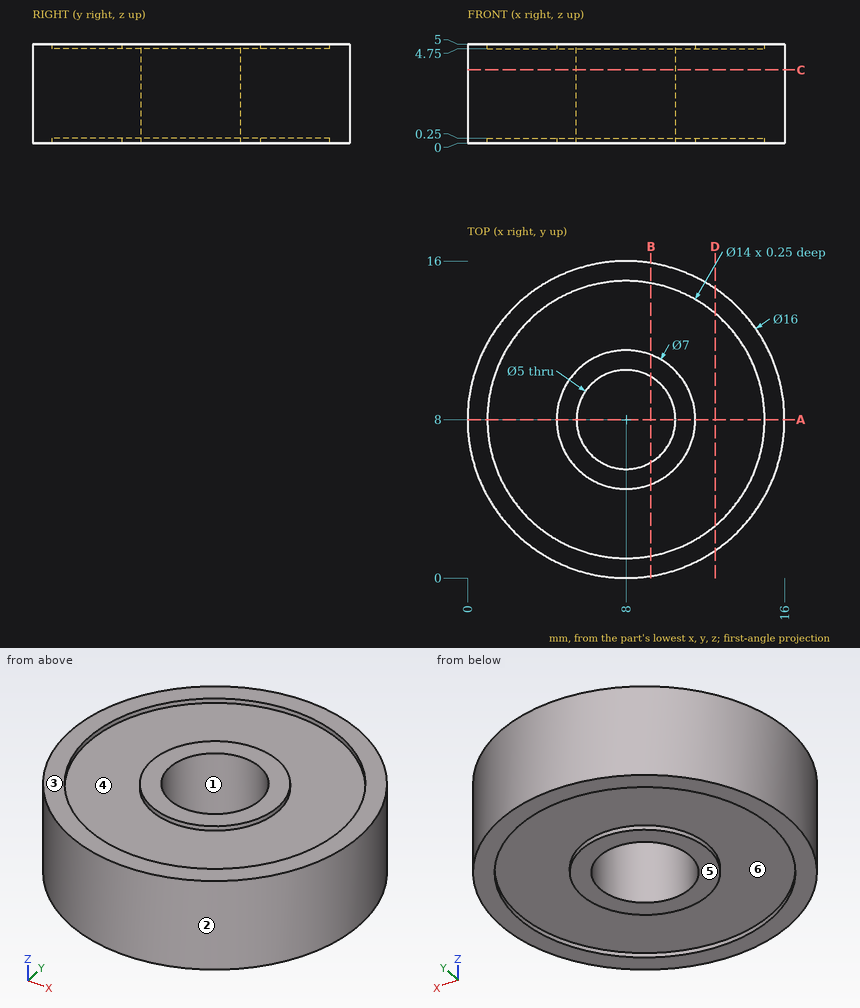
The figure shows three views and two pictorial views of one solid part (mm, origin at its lowest corner). Answer the questions. A direction names the side the tool comes from. Coordinates: 2 decimals unless noted, no trailing zeros. Order: outer loops, then holes, each group sorted by start corner. A loop starts at its lowest first (then second) coordinate and runs counter-clockwise, first axis right, second up. Notation, with made-up numbers: (-5.75, 16.5) - (20.25, 16.5) arc R16 ccw to (20.25, 20.5) - close; hole circle Ø8 at (-2.75, -23.75). An arc over 180 degrees is marked (long way). Answer as a JSON object with one key per item and string values.
1. Each of these flat-tipped pins is pushed along its axis until it touches: P1, Ø1.5, axis at x = 2.5, z = 0.5, coming from the +Y side; P2, Ø1, axis at x = 11.5, z = 0.5, coming from the -Y side. Where does it stop, or does it pass through?
Output values:
{"P1": "stops at y = 14.44", "P2": "stops at y = 0.58"}
2. Find section D-D on x = 12.5. Determine the outline of the cut face in (y, z), plus the area to 3 significant figures.
Output values:
{"outline": "(1.39, 0) - (2.64, 0) - (2.64, 0.25) - (13.36, 0.25) - (13.36, 0) - (14.61, 0) - (14.61, 5) - (13.36, 5) - (13.36, 4.75) - (2.64, 4.75) - (2.64, 5) - (1.39, 5) - close", "area": "60.8 mm²"}
3. Consider line 1 (X direction, y = 8, z = 0.1); line 2 (Y direction, x = 8, z = 2.9). Determine where each line is inside the solid, lowest interval first.
Output values:
{"line 1": "x = 0 to 1, 4.5 to 5.5, 10.5 to 11.5, 15 to 16", "line 2": "y = 0 to 5.5, 10.5 to 16"}
4. Find section A-A on y = 8. Determine the outline of the cut face in (x, z).
Output values:
{"outline": "(0, 0) - (1, 0) - (1, 0.25) - (4.5, 0.25) - (4.5, 0) - (5.5, 0) - (5.5, 5) - (4.5, 5) - (4.5, 4.75) - (1, 4.75) - (1, 5) - (0, 5) - close; (10.5, 0) - (11.5, 0) - (11.5, 0.25) - (15, 0.25) - (15, 0) - (16, 0) - (16, 5) - (15, 5) - (15, 4.75) - (11.5, 4.75) - (11.5, 5) - (10.5, 5) - close"}
5. The mould has two halves that part along X. Classify the marked faces 1, 2, 3 and 4: +X half, -X half, draft (parallel to the pull), parting line (faces both ways), or undercut.
Output values:
{"face 1": "undercut", "face 2": "parting line", "face 3": "draft", "face 4": "undercut"}
6. Find section B-B on x = 9.25. Determine the outline of the cut face in (y, z).
Output values:
{"outline": "(0.1, 0) - (1.11, 0) - (1.11, 0.25) - (4.73, 0.25) - (4.73, 0) - (5.83, 0) - (5.83, 5) - (4.73, 5) - (4.73, 4.75) - (1.11, 4.75) - (1.11, 5) - (0.1, 5) - close; (10.17, 0) - (11.27, 0) - (11.27, 0.25) - (14.89, 0.25) - (14.89, 0) - (15.9, 0) - (15.9, 5) - (14.89, 5) - (14.89, 4.75) - (11.27, 4.75) - (11.27, 5) - (10.17, 5) - close"}
7. Find section C-C on z = 3.7. Determine the outline of the cut face in (x, y).
Output values:
{"outline": "circle Ø16 at (8, 8); hole circle Ø5 at (8, 8)"}
8. A tool of negligible diameter and unlimited length cuts with its end or side. For the marked faces 5 and 6, from which of +Z, -Z, +X, -X, +Y, -Y can it reach the whole face along a straight path? Write none if from no direction.
Output values:
{"face 5": "-Z, +X, -X, +Y, -Y", "face 6": "-Z"}
